Autodesk Inventor part; units mm, degrees
ref_plane "YZ Plane" through (0, 0, 0) normal (1, 0, 0) x (0, 1, 0)
ref_plane "XZ Plane" through (0, 0, 0) normal (0, 1, 0) x (-1, 0, 0)
ref_plane "XY Plane" through (0, 0, 0) normal (0, 0, 1) x (1, 0, 0)
sketch "Sketch1" plane through (0, 0, 0) normal (0, 1, 0) x (-1, 0, 0)
  line L0 (70.8919, 46.3756) -> (99.3426, 56.8576)
  line L1 (24.7543, -14.1235) -> (48.4088, 27.336)
  line L2 (-28.5, 146) -> (-28.5, 0)
  line L3 (51.0145, 25.8493) -> (27.3601, -15.6101)
  line L4 (100.3797, 54.0426) -> (71.929, 43.5606)
  line L5 (-31.5, 0) -> (-31.5, 146)
  arc A0 (99.3426, 56.8576) -> (-28.5, 146) centre (66.5, 146) ccw
  arc A1 (70.8919, 46.3756) -> (48.4088, 27.336) centre (85.7575, 6.0269) ccw
  arc A2 (-28.5, 0) -> (24.7543, -14.1235) centre (0, 0) ccw
  arc A3 (-31.5, 0) -> (27.3601, -15.6101) centre (0, 0) ccw
  arc A4 (71.929, 43.5606) -> (51.0145, 25.8493) centre (85.7575, 6.0269) ccw
  arc A5 (100.3797, 54.0426) -> (-31.5, 146) centre (66.5, 146) ccw
  dimension "d0" = 95
  dimension "d1" = 40
  dimension "d2" = 28.5
  dimension "d3" = 31.5
  dimension "d4" = 146
  dimension "d5" = 146
  dimension "d6" = 98
  dimension "d7" = 95
  dimension "d8" = 146
  dimension "d9" = 66.5
  dimension "d10" = 47.7328
  dimension "d11" = 53.2544
  dimension "d12" = 43
  dimension "d13" = 58.8601
  dimension "d14" = 47.7328
  dimension "d15" = 91.9574
  dimension "d16" = 139.9731
  dimension "d17" = 85.7575
  dimension "d18" = 150.293
  dimension "d19" = 0
  dimension "d20" = 0
extrude "Extrusion1" add sketch "Sketch1" along normal blind 20
properties part number "50-01-001"
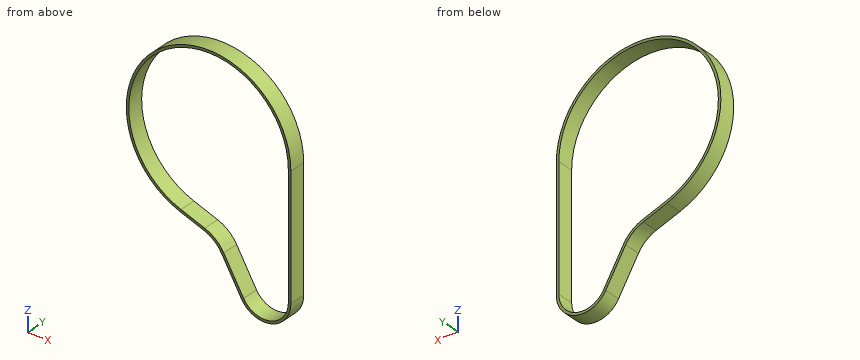
Geometry: final body of the model. Coordinates: model frame, mm. Give positions to 0.01 mm unless a question says otherwise; leave off trailing zeros. Order: outer loops, then holes, each group sorted by start corner. A loop starts at its lowest first (then second) coordinate and runs counter-clockwise, first axis right, second up. Notation, with made-up numbers: (42.25, 70.25) -> (48.25, 70.25) arc R16 ccw to (48.25, 74.25) -> close; hole circle Ø10 at (7, -5.75). An arc over 180 degrees is marked (long way). Write each question's results on one line, items separated by ' | '.
1) Cut plane A-A (y = 3.5). Output: boundary loops of the cut face in (x, z), and give its area (3 significant figures).
Geometry says:
outline: (-100.38, 54.04) -> (-71.93, 43.56) arc R40 cw to (-51.01, 25.85) -> (-27.36, -15.61) arc R31.5 ccw to (31.5, 0) -> (31.5, 146) arc R98 ccw (long way) to start; hole (-99.34, 56.86) -> (-70.89, 46.38) arc R43 cw to (-48.41, 27.34) -> (-24.75, -14.12) arc R28.5 ccw to (28.5, 0) -> (28.5, 146) arc R95 ccw (long way) to start | area: 2,260 mm²
2) First-contact query: pin 1 Ø2 at (x, y) = (3, 16) entering from -Z; pin 2 Ø1.5 at (x, y) = (-77, 12.5) entering from +Z; pin 3 Ø4 at (y, z) = (14, 54) entering from -X. Flat tips, straight axial feed; report the tip coordinate or a pass-through.
Geometry says:
pin 1: stops at z = -31.44 | pin 2: stops at z = 243.51 | pin 3: stops at x = -105.28
3) Cut plane C-C (x = -58). Output: boundary loops of the cut face in (y, z).
Geometry says:
outline: (0, 34.83) -> (20, 34.83) -> (20, 38.87) -> (0, 38.87) -> close; (0, 240.62) -> (20, 240.62) -> (20, 243.63) -> (0, 243.63) -> close
4) Cut plane B-B (z = 18.5). Output: boundary loops of the cut face in (x, y).
Geometry says:
outline: (-46.82, 0) -> (-43.37, 0) -> (-43.37, 20) -> (-46.82, 20) -> close; (28.5, 0) -> (31.5, 0) -> (31.5, 20) -> (28.5, 20) -> close
5) Line query: line 1 along Z through (x, y) = (9, 4.5); line 2 along Z through (x, y) = (8, 2.75); line 3 along X through (y, z) = (7.5, 139). Output: solid intervals per line, ascending.
Geometry says:
line 1: z = -30.19 to -27.04, 203.66 to 208.48 | line 2: z = -30.47 to -27.35, 204.95 to 209.67 | line 3: x = -164.25 to -161.24, 28.5 to 31.5
